Read the model definition and answer for the solid it produces. Units are mm, in the model's axes. Face numbers are marked on the shaded views. A direction names the side the tool comes from. Coordinates: 2 decimals unless noted, no trailing zeros. Loops run counter-clockwise (first coordinate to the right, second up) from the corner with the lowest first, then second, coordinate; pieces in that order, holes last. Notation, with made-up numbers: (89.5, -23.75) - (147.5, -23.75) arc R14 ccw to (147.5, -11.75) - close; hole circle Ø3 at (66, 5.5). An arc over 180 degrees is marked (long way). Use one line per item in the form item = value.
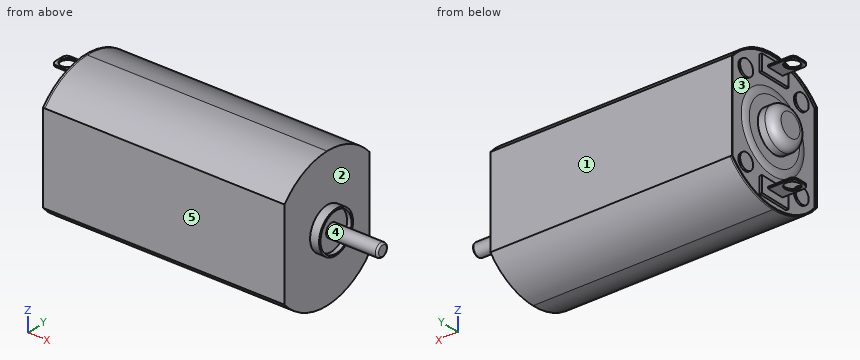
from build123d import *

# Parameters (mm, degrees)
EXTRUDE_1_DEPTH     = 26.8
EXTRUDE_START       = -0.2
EXTRUDE_1_2_DEPTH   = 0.2
SKETCH_2_R          = 4.35
EXTRUDE_2_DEPTH     = 0.2
FILLET_1_R          = 2
SKETCH_3_R          = 2.3
EXTRUDE_3_DEPTH     = 1.8
FILLET_2_R          = 1
SKETCH_4_W          = 1.8
SKETCH_4_H          = 3.7
EXTRUDE_8_DEPTH     = 0.3
SKETCH_4_4_W        = 0.2
SKETCH_4_4_H        = 2
EXTRUDE_9_DEPTH     = 3.2
CUT_EXTRUDE_1_REACH = 32.784
SKETCH_5_R          = 0.8
CUT_EXTRUDE_2_REACH = 32.784
SKETCH_6_R          = 0.8
FILLET_3_R          = 0.5
SKETCH_7_R          = 0.9
EXTRUDE_10_DEPTH    = 0.2
SKETCH_8_R          = 2.35
SKETCH_8_R_2        = 2.15
EXTRUDE_2_2_DEPTH   = 1
SKETCH_8_2_R        = 2.35
EXTRUDE_11_DEPTH    = 0.5
SKETCH_9_R          = 0.75
EXTRUDE_12_DEPTH    = 6.2
FILLET_4_R          = 0.2


# Read off the part's stored shape, not the designer's step: 拉伸-薄壁1
with BuildPart() as part:
    # 草图1 → Extrude 1 (new body)
    with BuildSketch(Plane(origin=(0, 0, 0), x_dir=(0, 0, -1), z_dir=(1, 0, 0))):
        with BuildLine():
            ThreePointArc((-7.75, 0), (-7.035897095, -3.249407956), (-5.025186564, -5.9))
            Line((-5.025186564, -5.9), (5.025186564, -5.9))
            ThreePointArc((5.025186564, -5.9), (7.035897095, -3.249407956), (7.75, 0))
            ThreePointArc((7.75, 0), (7.035897095, 3.249407956), (5.025186564, 5.9))
            Line((5.025186564, 5.9), (-5.025186564, 5.9))
            ThreePointArc((-5.025186564, 5.9), (-7.035897095, 3.249407956), (-7.75, 0))
        make_face()
    extrude(amount=EXTRUDE_1_DEPTH)



with BuildPart() as body_2:
    # Extrude 1 2 outline → Extrude 1 2 (new body)
    with BuildSketch(Plane(origin=(0, 0, 0), x_dir=(0, 0, -1), z_dir=(1, 0, 0)).offset(EXTRUDE_START)):
        with BuildLine():
            Line((5.025186564, 5.9), (-5.025186564, 5.9))
            ThreePointArc((-5.025186564, 5.9), (-7.75, 0), (-5.025186564, -5.9))
            Line((-5.025186564, -5.9), (5.025186564, -5.9))
            ThreePointArc((5.025186564, -5.9), (7.75, 0), (5.025186564, 5.9))
        make_face()
        with BuildLine():
            ThreePointArc((-4.988236161, -5.8), (-7.65, 0), (-4.988236161, 5.8))
            Line((-4.988236161, 5.8), (4.988236161, 5.8))
            ThreePointArc((4.988236161, 5.8), (7.65, 0), (4.988236161, -5.8))
            Line((4.988236161, -5.8), (-4.988236161, -5.8))
        make_face(mode=Mode.SUBTRACT)
    extrude(amount=EXTRUDE_1_2_DEPTH)


with BuildPart() as part_1:
    add(part.part)

    add(body_2.part)  # Extrude 2 merges body 2
    # 草图2 → Extrude 2 (add)
    with BuildSketch(Plane.ZY):
        Circle(SKETCH_2_R)
    extrude(amount=EXTRUDE_2_DEPTH)

    # 圆角1
    # the kernel refuses this fillet: 2 mm, written as the material it takes off along each edge
    with BuildSketch(Plane(origin=(-0.2, 0, 0), x_dir=(0, 0, 1), z_dir=(0, -1, 0))) as fillet_1_piece_1:
        with BuildLine():
            CenterArc((3.478220211, -2), FILLET_1_R, 64.158067237, 25.841932763)
            Line((3.478220211, 0), (3.478220211, 0.04))
            Line((3.478220211, 0.04), (4.35, 0.04))
            Line((4.35, 0.04), (4.39, 0))
            ThreePointArc((4.39, 0), (4.39, -0.1), (4.367435596, -0.164))
            Line((4.367435596, -0.164), (4.35, -0.2))
        make_face()
    revolve(axis=Axis((-0.2, 0, 0), (-1, 0, 0)), mode=Mode.SUBTRACT)

    # 草图3 → 凸台-拉伸3 (add)
    with BuildSketch(Plane.ZY.offset(0.2)):
        Circle(SKETCH_3_R)
    extrude(amount=EXTRUDE_3_DEPTH)

    # 圆角2
    fillet_2_edges = [part_1.edges().sort_by_distance(p)[0] for p in [
        (-2, 0, -2.3),
    ]]
    fillet(fillet_2_edges, radius=FILLET_2_R)

    # 草图4 → 凸台-拉伸8 (add)
    with BuildSketch(Plane.ZY):
        with Locations((-6.1, 0)):
            Rectangle(SKETCH_4_W, SKETCH_4_H)
        with Locations((6.1, 0)):
            Rectangle(SKETCH_4_W, SKETCH_4_H)
    extrude(amount=EXTRUDE_8_DEPTH)

    # 草图4<4> → 凸台-拉伸9 (add)
    with BuildSketch(Plane.ZY):
        with Locations((6.1, 0)):
            Rectangle(SKETCH_4_4_W, SKETCH_4_4_H)
        with Locations((-6.1, 0)):
            Rectangle(SKETCH_4_4_W, SKETCH_4_4_H)
    extrude(amount=EXTRUDE_9_DEPTH)

    # 草图5 → 切除-拉伸1 (cut, up to next)
    with BuildSketch(Plane(origin=(0, 0, -6.2), x_dir=(-1, 0, 0), z_dir=(0, 0, -1)), mode=Mode.PRIVATE) as cut_extrude_1_sk1:
        with Locations((2.2, 0)):
            Circle(SKETCH_5_R)
    cut_extrude_1_tool1 = extrude(cut_extrude_1_sk1.sketch, amount=-CUT_EXTRUDE_1_REACH, mode=Mode.PRIVATE) & part_1.part
    add(cut_extrude_1_tool1.solids().sort_by_distance((-2.2, 0, -6.2))[0], mode=Mode.SUBTRACT)

    # 草图6 → 切除-拉伸2 (cut, up to next)
    with BuildSketch(Plane.XY.offset(6.2), mode=Mode.PRIVATE) as cut_extrude_2_sk1:
        with Locations(Location((-2.2, 0, 0), (0, 0, 180))):
            Circle(SKETCH_6_R)
    cut_extrude_2_tool1 = extrude(cut_extrude_2_sk1.sketch, amount=-CUT_EXTRUDE_2_REACH, mode=Mode.PRIVATE) & part_1.part
    add(cut_extrude_2_tool1.solids().sort_by_distance((-2.2, 0, 6.2))[0], mode=Mode.SUBTRACT)

    # 圆角3
    fillet_3_edges = [part_1.edges().sort_by_distance(p)[0] for p in [
        (-3.2, -1, -6.1),
        (-3.2, 1, -6.1),
        (-3.2, 1, 6.1),
        (-3.2, -1, 6.1),
    ]]
    fillet(fillet_3_edges, radius=FILLET_3_R)

    # 草图7 → 凸台-拉伸10 (add)
    with BuildSketch(Plane.ZY):
        with Locations(Location((-4.7, 3.85, 0), (0, 0, 180))):
            Circle(SKETCH_7_R)
        with Locations(Location((4.7, 3.85, 0), (0, 0, 180))):
            Circle(SKETCH_7_R)
        with Locations(Location((4.7, -3.85, 0), (0, 0, 180))):
            Circle(SKETCH_7_R)
        with Locations(Location((-4.7, -3.85, 0), (0, 0, 180))):
            Circle(SKETCH_7_R)
    extrude(amount=EXTRUDE_10_DEPTH)

    # 草图8 → Extrude 2 2 (add)
    with BuildSketch(Plane(origin=(26.8, 0, 0), x_dir=(0, 0, -1), z_dir=(1, 0, 0))):
        Circle(SKETCH_8_R)
        Circle(SKETCH_8_R_2, mode=Mode.SUBTRACT)
    extrude(amount=EXTRUDE_2_2_DEPTH)

    # 草图8<2> → 凸台-拉伸11 (add)
    with BuildSketch(Plane(origin=(26.8, 0, 0), x_dir=(0, 0, -1), z_dir=(1, 0, 0))):
        Circle(SKETCH_8_2_R)
    extrude(amount=EXTRUDE_11_DEPTH)

    # 草图9 → 凸台-拉伸12 (add)
    with BuildSketch(Plane(origin=(26.8, 0, 0), x_dir=(0, 0, -1), z_dir=(1, 0, 0))):
        with Locations(Location((0, 0, 0), (0, 0, 180))):
            Circle(SKETCH_9_R)
    extrude(amount=EXTRUDE_12_DEPTH)

    # 圆角4
    fillet_4_edges = [part_1.edges().sort_by_distance(p)[0] for p in [
        (33, 0, -0.75),
    ]]
    fillet(fillet_4_edges, radius=FILLET_4_R)


solid = part_1.part
Item 1: Find the intervals of material crossed by L1, parallel to Y at x = -2.2, z = -6.1; L2, parallel to X at y = 3.5, z = -6.5; L3, parallel to Z at x = 15.5, y = 1.25, in increasing order.
Results below:
L1 = -1 to -0.8, 0.8 to 1
L2 = 0 to 26.8
L3 = -7.65 to 7.65
Item 2: For a pull along Y with two mould halves and no side action, classify the marked faces 1, 2 and 3 as +Y half, -Y half, draft (parallel to the pull), parting line (faces both ways), or undercut.
Results below:
face_1 = +Y half
face_2 = draft
face_3 = undercut
Item 3: The part is cut by section B-B on x = 10.5. Give the vertices of the cut face in (y, z), plus the area to 3 significant figures.
Results below:
outline = (-5.9, -5.03) arc R7.75 ccw to (5.9, -5.03) - (5.9, 5.03) arc R7.75 ccw to (-5.9, 5.03) - close
area = 163 mm²
Item 4: The part is cut by section A-A on x = 29.5. Give the vertices of the cut face in (y, z), plus the area to 3 significant figures.
Results below:
outline = circle Ø1.5 at (0, 0)
area = 1.77 mm²
Item 5: Which of the six approach directions +Z, -Z, +X, -X, +Y, -Y give full straight-line access (tool end or side, diameter ignored) to the marked faces 4 and 5?
Results below:
face_4 = +X
face_5 = +Z, -Z, +X, -X, -Y
Item 6: Each of these flat-tipped pins is pushed along its axis until it touches: P1, Ø2, axis at y = 4, z = -5, coming from the -X side; P2, Ø1.3, axis at y = 0.5, z = 0, coming from the -X side; P3, Ø5, axis at x = 11, y = 4.5, coming from the -Z side. Where does it stop, or does it pass through?
Results below:
P1 = -0.2
P2 = -2
P3 = -7.49
